from build123d import *

# Parameters (mm, degrees)
F1_DEPTH = 25.4
F2_R     = 12.69999
F3_R     = 6.35
F4_DEPTH = 50.8
F5_R     = 12.69999
F6_R     = 6.35
F8_DEPTH = 25.4


# Not quite as in the source:
# - a fillet or chamfer is up to 0.001 mm smaller than in the source, because OpenCascade refuses the exact size


with BuildPart() as f1:
    # F0 (on Front) → F1 (new body)
    with BuildSketch(Plane.XZ):
        Polygon((0, 38.1), (0, 0), (76.2, 0), (76.2, 12.7), (25.4, 12.7), (25.4, 38.1), align=None)
    extrude(amount=F1_DEPTH)

    # F2 (radius 12.7 in the source; OpenCascade refuses exactly that, so slightly less here)
    f2_edges = [f1.edges().sort_by_distance(p)[0] for p in [
        (25.4, 0, 25.4),
        (25.4, -25.4, 25.4),
        (0, -25.4, 19.05),
        (0, 0, 19.05),
    ]]
    fillet(f2_edges, radius=F2_R)

    # F3 (on face) → F4 (cut)
    with BuildSketch(Plane.XY.offset(38.1)):
        with Locations((12.7, -12.7)):
            Circle(F3_R)
    extrude(amount=-F4_DEPTH, mode=Mode.SUBTRACT)

    # F5 (radius 12.7 in the source; OpenCascade refuses exactly that, so slightly less here)
    f5_edges = [f1.edges().sort_by_distance(p)[0] for p in [
        (76.2, 0, 6.35),
        (76.2, -25.4, 6.35),
    ]]
    fillet(f5_edges, radius=F5_R)

    # F6 (on face) + F7 (on face) → F8 (cut)
    with BuildSketch(Plane.XY.offset(12.7)):
        with Locations((38.1, -12.7)):
            Circle(F6_R)
    with BuildSketch(Plane.XY.offset(12.7)):
        with BuildLine():
            Line((40.7903380557, -18.4519197792), (60.8096619443, -18.4519197792))
            ThreePointArc((60.8096619443, -18.4519197792), (57.2698982045, -11.4718584702), (63.1938608334, -6.3573839143))
            Line((63.1938608334, -6.3573839143), (38.4061391666, -6.3573839143))
            ThreePointArc((38.4061391666, -6.3573839143), (42.6970905858, -8.3194454522), (44.45, -12.7))
            ThreePointArc((44.45, -12.7), (43.4575249254, -16.108728014), (40.7903380557, -18.4519197792))
        make_face()
        with BuildLine():
            ThreePointArc((63.1938608334, -6.3573839143), (57.2698982045, -11.4718584702), (60.8096619443, -18.4519197792))
            ThreePointArc((60.8096619443, -18.4519197792), (66.908728014, -18.0575249254), (69.85, -12.7))
            ThreePointArc((69.85, -12.7), (68.0970905858, -8.3194454522), (63.8061391666, -6.3573839143))
            Line((63.8061391666, -6.3573839143), (63.1938608334, -6.3573839143))
        make_face()
    extrude(amount=-F8_DEPTH, mode=Mode.SUBTRACT)


solid = f1.part
The model under review builds one solid part; all positions refer to its coordinate system, in mm. A direction names the side the tool comes from. Give positions to 0.01 mm unless a question says otherwise; leave off trailing zeros. Write each loop counter-clockwise with the first axis right and the second up, starting at its lowest first coordinate (ties: lowest second). Pieces come first, ordered by that corner, then holes.
1. Add section D-D, the plane z = 4. Count the separate pieces of the cut face and the enclosed holes in it, plus the area to 3 significant figures.
2. Wall thickness on L1, parallel to Y at x = 43, z = 12; L2, parallel to Y at x = 38.1, z = 9; L3, parallel to Z at x = 39, y = -4: over which ranges is each line inside the solid? List them lowest first.
3. For P1, Ø2, axis at x = 56, y = -18.5, coming from the +Z side; P2, Ø8, axis at y = -8.5, z = 32.5, coming from the +X side, all flat-tipped, find the tip position at first contact; note any pin that passes through.
4. Add section A-A, the plane x = 58. Write out the cut boundary in (y, z), plus the area to 3 significant figures.
5. Draft analysis for pull direction Y (two halves, no side actions). For faces 4 (the flat face through (19, -15, 38.1)), 5 (the cylindrical face through (21.78, -21.58, 25.58)), 6 (the cylindrical face through (31.84, -13.77, 6.44)), state which applies: +Y half, -Y half, draft (parallel to the pull), parting line (faces both ways), or undercut.
6. Add section C-C, the plane y = -9. Write out the cut boundary in (x, z), plus the area to 3 significant figures.
7. Tool access review of faces 1 (the cylindrical face through (21.78, -3.82, 25.58)), 2 (the flat face through (51, -18.452, 6)), 3 (the flat face through (38, 0, 8)): name each direction out of +Z, -Z, +X, -X, +Y, -Y from which nothing blocks a thin tool from reaching the whole face with its end or side.
Worked answers:
1. separate pieces: 1
1. enclosed holes: 2
1. area: 1,230 mm2
2. L1: y = -25.4 to -18.45, -6.36 to 0
2. L2: y = -25.4 to -19.05, -6.35 to 0
2. L3: z = 0 to 12.7
3. P1: stops at z = 12.7
3. P2: stops at x = 25.4
4. outline: (-25.4, 0) - (-18.45, 0) - (-18.45, 12.7) - (-25.4, 12.7) - close; (-6.36, 0) - (0, 0) - (0, 12.7) - (-6.36, 12.7) - close
4. area: 169 mm2
5. face 4: draft
5. face 5: -Y half
5. face 6: undercut
6. outline: (0.55, 0) - (7.54, 0) - (7.54, 38.1) - (0.55, 38.1) - close; (17.86, 0) - (32.94, 0) - (32.94, 12.7) - (24.85, 12.7) - (24.85, 38.1) - (17.86, 38.1) - close; (68.66, 0) - (75.65, 0) - (75.65, 12.7) - (68.66, 12.7) - close
6. area: 724 mm2
7. face 1: +Z, +X, +Y
7. face 2: +Z, -Z
7. face 3: +Z, -Z, +X, -X, +Y
